Job drawing, mm, ordinate dimensions from the low corner. One solid piece. A direction names the side the tool comes from. Round coordinates to 2 decimals unless told otherwise and drop trailing zeros. Loops run counter-clockwise (first coordinate to the right, second up) from the corner with the lowest first, then second, coordinate; pieces in that order, holes last. Notation, with made-up numbers: M 47.5,63.25 L 72.5,63.25 A12 ccw 72.5,78.25 Z; hole C 17,72.5 d6. An arc over 180 degrees is marked long. Write each question's results on one line, items separated by ' | '. Start each with the question number.
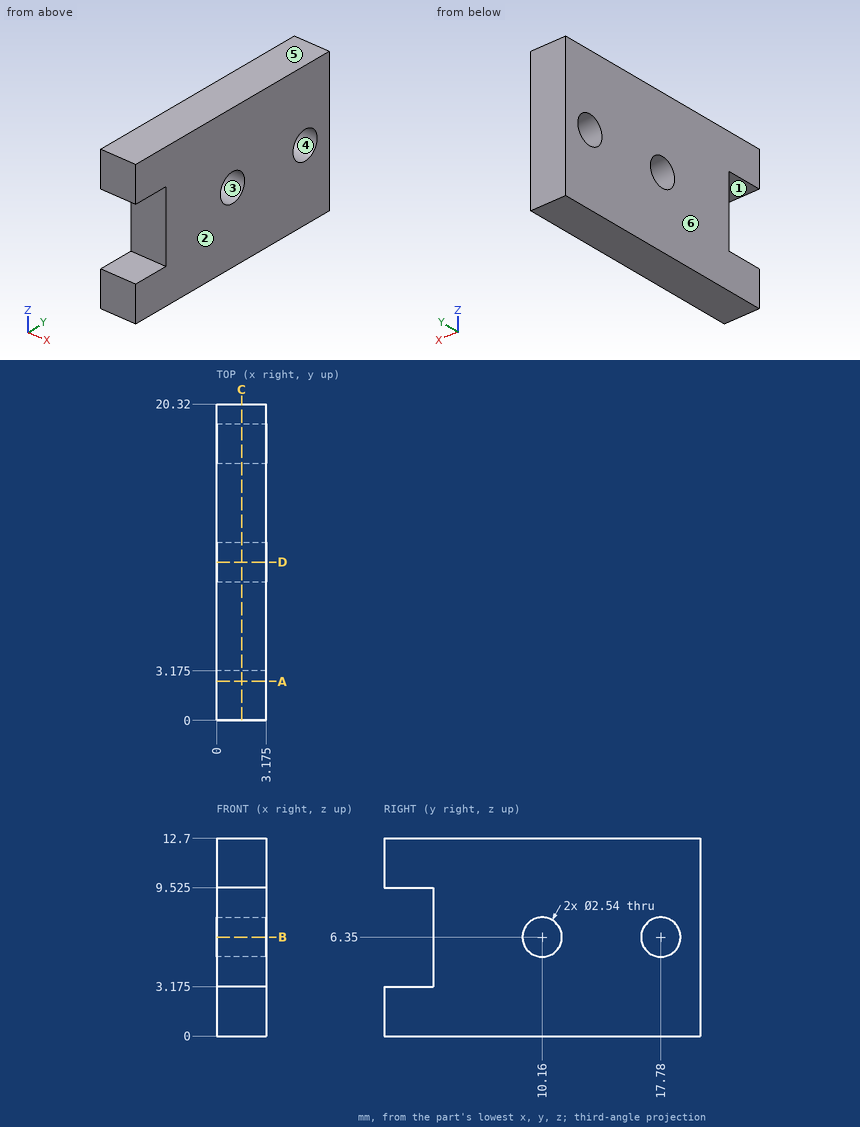
Item 1: Saw through at B-B, the plane z = 6.35. Give the cut face in (x, y) (3 decimals).
Item 2: Drill centre lines: line 1 along Y through (x, z) = (1.5, 6.35) (3 decimals); line 2 along Z through (x, y) = (0.55, 1.75) (3 decimals); line 3 along Y through (x, z) = (0.8, 6.75) (3 decimals). Where is each one in solid material? Low to high. Write a range as [from, to].
Item 3: Tool access for the marked faces 1 and 2: list every direction of +Z, -Z, +X, -X, +Y, -Y with a clear straight run to the whole face (end or side of a thin tool).
Item 4: Drop flat-ended pins along their axis: pin 1 (1.5 mm diameter, centred on y = 17, z = 2.5, fed in from -X); pin 2 (1 mm diameter, centred on x = 2, z = 7, fed in from -Y) (3 decimals). Give the stop position or say it passes through.
Item 5: Mould opens along Z. For the marked faces 3, 4, 5 and 6 say: released by +Z, released by -Z, zero draft, split by the parting line, or undercut.
Item 6: Saw through at D-D, the plane y = 10.16. Give the cut face in (x, z) (3 decimals).
Item 7: Saw through at A-A, the plane y = 2.5. Give the cut face in (x, z) (3 decimals), then the cut area to 3 significant figures.
Item 8: Saw through at C-C, the plane x = 1.6. Give the cut face in (y, z) (3 decimals), then the cut area to 3 significant figures.
Working result:
1) outline: M 0,3.175 L 3.175,3.175 L 3.175,8.89 L 0,8.89 Z; M 0,11.43 L 3.175,11.43 L 3.175,16.51 L 0,16.51 Z; M 0,19.05 L 3.175,19.05 L 3.175,20.32 L 0,20.32 Z
2) line 1: y = [3.175, 8.89], [11.43, 16.51], [19.05, 20.32] | line 2: z = [0, 3.175], [9.525, 12.7] | line 3: y = [3.175, 8.955], [11.365, 16.575], [18.985, 20.32]
3) face 1: +X, -X, -Y | face 2: +Z, -Z, +X, +Y, -Y
4) pin 1: stops at x = 0 | pin 2: stops at y = 3.175
5) face 3: undercut | face 4: undercut | face 5: released by +Z | face 6: zero draft
6) outline: M 0,0 L 3.175,0 L 3.175,5.08 L 0,5.08 Z; M 0,7.62 L 3.175,7.62 L 3.175,12.7 L 0,12.7 Z
7) outline: M 0,0 L 3.175,0 L 3.175,3.175 L 0,3.175 Z; M 0,9.525 L 3.175,9.525 L 3.175,12.7 L 0,12.7 Z | area: 20.2 mm²
8) outline: M 0,0 L 20.32,0 L 20.32,12.7 L 0,12.7 L 0,9.525 L 3.175,9.525 L 3.175,3.175 L 0,3.175 Z; hole C 10.16,6.35 d2.54; hole C 17.78,6.35 d2.54 | area: 228 mm²
